Verification items for the finished model (mm, model axes). Face numbers are marked on the shaded views. A direction names the side the tool comes from. Round coordinates to 2 decimals unless told otherwise and drop trailing zeros. Order: outer loops, then holes, each group sorted by start corner. A loop starts at its lowest first (then second) coordinate and runs counter-clockwise, first axis right, second up. Notation, with made-up numbers: (73, -31.75) -> (113, -31.75) arc R17 ccw to (113, 0.25) -> close; hole circle Ø9 at (12, 82.25). An arc over 180 degrees is marked (long way). Answer in a Markdown table with one row per item. Add a question column.
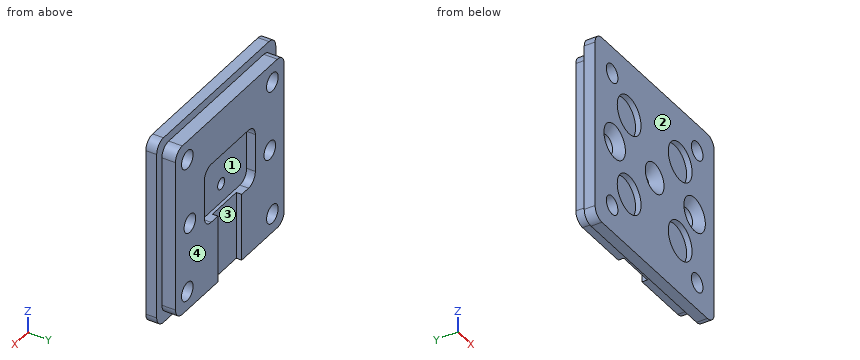
```python
from build123d import *

# Parameters (mm, degrees)
EXTRUDE_1_DEPTH              = 2.5
EXTRUDE_2_DEPTH              = 2
HOLE_WIZARD_3_4_D            = 3.4
CUT_EXTRUDE_2193_DEPTH       = 1.6
HOLE_WIZARD_3_D              = 3.4
HOLE_WIZARD_3_CSINK_D        = 6.3
HOLE_WIZARD_3_CSINK_ANGLE    = 90
SKETCH_8_W                   = 7
SKETCH_8_H                   = 12.475
CUT_EXTRUDE_3485_DEPTH       = 1
SKETCH_11_R                  = 3.5
CUT_EXTRUDE_7_1_DEPTH        = 1
HOLE_WIZARD_M2_5_D           = 2.05
HOLE_WIZARD_M2_5_CSINK_D     = 5.5
HOLE_WIZARD_M2_5_CSINK_ANGLE = 90


with BuildPart() as part:
    # Эскиз1 → Бобышка-Вытянуть1 (new body)
    with BuildSketch(Plane(origin=(0, 0, 0), x_dir=(1, 0, 0), z_dir=(0, 1, 0))):
        with BuildLine():
            Line((-13.975, 15.975), (13.975, 15.975))
            ThreePointArc((13.975, 15.975), (15.389213562, 15.389213562), (15.975, 13.975))
            Line((15.975, 13.975), (15.975, -13.975))
            ThreePointArc((15.975, -13.975), (15.389213562, -15.389213562), (13.975, -15.975))
            Line((13.975, -15.975), (-13.975, -15.975))
            ThreePointArc((-13.975, -15.975), (-15.389213562, -15.389213562), (-15.975, -13.975))
            Line((-15.975, -13.975), (-15.975, 13.975))
            ThreePointArc((-15.975, 13.975), (-15.389213562, 15.389213562), (-13.975, 15.975))
        make_face()
    extrude(amount=EXTRUDE_1_DEPTH)

    # Эскиз9 → Бобышка-Вытянуть2 (add)
    with BuildSketch(Plane.XZ):
        with BuildLine():
            Line((-15.5, 17.5), (15.5, 17.5))
            ThreePointArc((15.5, 17.5), (16.914213562, 16.914213562), (17.5, 15.5))
            Line((17.5, 15.5), (17.5, -15.5))
            ThreePointArc((17.5, -15.5), (16.914213562, -16.914213562), (15.5, -17.5))
            Line((15.5, -17.5), (-15.5, -17.5))
            ThreePointArc((-15.5, -17.5), (-16.914213562, -16.914213562), (-17.5, -15.5))
            Line((-17.5, -15.5), (-17.5, 15.5))
            ThreePointArc((-17.5, 15.5), (-16.914213562, 16.914213562), (-15.5, 17.5))
        make_face()
    extrude(amount=EXTRUDE_2_DEPTH)

    # Диаметр отверстия Ø3.4 (through all)
    with Locations(Plane.XZ.offset(2)):
        with Locations((-12.5, -12.5), (12.5, -12.5), (12.5, 12.5), (-12.5, 12.5)):
            Hole(HOLE_WIZARD_3_4_D / 2)

    # Эскиз4 → Cut-Extrude 2193 (cut)
    with BuildSketch(Plane(origin=(0, 2.5, 0), x_dir=(1, 0, 0), z_dir=(0, 1, 0))):
        with BuildLine():
            Line((-5.5, 3.5), (5.5, 3.5))
            ThreePointArc((5.5, 3.5), (6.914213562, 2.914213562), (7.5, 1.5))
            Line((7.5, 1.5), (7.5, -5.5))
            ThreePointArc((7.5, -5.5), (6.914213562, -6.914213562), (5.5, -7.5))
            Line((5.5, -7.5), (-5.5, -7.5))
            ThreePointArc((-5.5, -7.5), (-6.914213562, -6.914213562), (-7.5, -5.5))
            Line((-7.5, -5.5), (-7.5, 1.5))
            ThreePointArc((-7.5, 1.5), (-6.914213562, 2.914213562), (-5.5, 3.5))
        make_face()
    extrude(amount=-CUT_EXTRUDE_2193_DEPTH, mode=Mode.SUBTRACT)

    # Крепление дна М3 (through all)
    with Locations(Plane(origin=(0, -2, 0), x_dir=(-1, 0, 0), z_dir=(0, -1, 0))):
        with Locations((11.75, 0), (-11.75, 0)):
            CounterSinkHole(HOLE_WIZARD_3_D / 2, HOLE_WIZARD_3_CSINK_D / 2, counter_sink_angle=HOLE_WIZARD_3_CSINK_ANGLE)

    # Эскиз8 → Cut-Extrude 3485 (cut)
    with BuildSketch(Plane(origin=(0, 2.5, 0), x_dir=(1, 0, 0), z_dir=(0, 1, 0))):
        with Locations((0, 9.7375)):
            Rectangle(SKETCH_8_W, SKETCH_8_H)
    extrude(amount=-CUT_EXTRUDE_3485_DEPTH, mode=Mode.SUBTRACT)

    # Эскиз11 → Вырез магнитов 7*1 (cut)
    with BuildSketch(Plane.XZ.offset(2)):
        with Locations(Location((-7.5, 7.5, 0), (0, 0, 270))):
            Circle(SKETCH_11_R)
        with Locations(Location((7.5, 7.5, 0), (0, 0, 270))):
            Circle(SKETCH_11_R)
        with Locations(Location((-7.5, -7.5, 0), (0, 0, 270))):
            Circle(SKETCH_11_R)
        with Locations(Location((7.5, -7.5, 0), (0, 0, 270))):
            Circle(SKETCH_11_R)
    extrude(amount=-CUT_EXTRUDE_7_1_DEPTH, mode=Mode.SUBTRACT)

    # Отверстие для настройки M2.5 (through all)
    with Locations(Plane(origin=(0, -2, 0), x_dir=(-1, 0, 0), z_dir=(0, -1, 0))):
        with Locations((0, 0)):
            CounterSinkHole(HOLE_WIZARD_M2_5_D / 2, HOLE_WIZARD_M2_5_CSINK_D / 2, counter_sink_angle=HOLE_WIZARD_M2_5_CSINK_ANGLE)


solid = part.part
```
1) Cross-section at C-C, the plane z = -12.5. Record the boundary of the cut face in (x, y) (3 decimals).
2) Draft check along X on the marked faces 3 and 4. Enter one of: +X half, -X half, draft (parallel to the pull), parting line (faces both ways), or undercut.
3) Tool access check on the marked faces 1 and 2. Record the directions out of +Z, -Z, +X, -X, +Y, -Y that give a thin tool (end or side, any length) a straight path to the whole face; none if there is none.
4) Thickness scan on L1, parallel to X at y = -1.7, z = -7.5; L2, parallel to Z at x = 5, y = 1.1 (3 decimals); L3, parallel to X at y = -1.75, z = -4.5. Record the ranges inside material, lowest first. Write a range as [from, to].
5) Depth check by flat-ended pin: P1, Ø11, axis at x = -7.5, z = 7.5, coming from the -Y side; P2, Ø0.5, axis at y = 1.5, z = 3.5, coming from the +X side (3 decimals); P3, Ø0.8, axis at y = 2, z = 2, coming from the -X side (3 decimals); P4, Ø0.5, axis at x = -0.5, y = 2, coming from the -Z side. Enter the tip coordinate at first touch or a pass-through.
6) Cross-section at D-D, the plane x = 11.75. Record the boundary of the cut face in (y, z) (3 decimals), and give its area (3 significant figures).
7) Cross-section at A-A, the plane x = 0. Record the boundary of the cut face in (y, z) (3 decimals), and give its area (3 significant figures).
8) Cross-section at B-B, the plane y = -1.55. Give the number of separate pieces and of enclosed holes in the cut face, and give its area (3 significant figures).
Results below:
| question | item | result |
|---|---|---|
| 1 | outline | (-17.5, -2) -> (-14.2, -2) -> (-14.2, 2.5) -> (-15.975, 2.5) -> (-15.975, 0) -> (-17.5, 0) -> close; (-10.8, -2) -> (10.8, -2) -> (10.8, 2.5) -> (3.5, 2.5) -> (3.5, 1.5) -> (-3.5, 1.5) -> (-3.5, 2.5) -> (-10.8, 2.5) -> close; (14.2, -2) -> (17.5, -2) -> (17.5, 0) -> (15.975, 0) -> (15.975, 2.5) -> (14.2, 2.5) -> close |
| 2 | face 3 | undercut |
| 2 | face 4 | draft |
| 3 | face 1 | +Y |
| 3 | face 2 | +Z, -Z, +X, -X, -Y |
| 4 | L1 | [-17.5, -11], [-4, 4], [11, 17.5] |
| 4 | L2 | [-15.975, -3.5], [7.5, 15.975] |
| 4 | L3 | [-17.5, -9.3], [-5.7, 5.7], [9.3, 17.5] |
| 5 | P1 | y = -2 |
| 5 | P2 | x = 15.975 |
| 5 | P3 | x = -15.975 |
| 5 | P4 | z = 7.5 |
| 6 | outline | (-2, -17.5) -> (0, -17.5) -> (0, -15.975) -> (2.5, -15.975) -> (2.5, -14.026) -> (-2, -14.026) -> close; (-2, -10.974) -> (2.5, -10.974) -> (2.5, -1.7) -> (-0.55, -1.7) -> (-2, -3.15) -> close; (-2, 3.15) -> (-0.55, 1.7) -> (2.5, 1.7) -> (2.5, 10.974) -> (-2, 10.974) -> close; (-2, 14.026) -> (2.5, 14.026) -> (2.5, 15.975) -> (0, 15.975) -> (0, 17.5) -> (-2, 17.5) -> close |
| 6 | area | 105 mm² |
| 7 | outline | (-2, -17.5) -> (0, -17.5) -> (0, -15.975) -> (1.5, -15.975) -> (1.5, -3.5) -> (0.9, -3.5) -> (0.9, -1.025) -> (-0.275, -1.025) -> (-2, -2.75) -> close; (-2, 2.75) -> (-0.275, 1.025) -> (0.9, 1.025) -> (0.9, 7.5) -> (2.5, 7.5) -> (2.5, 15.975) -> (0, 15.975) -> (0, 17.5) -> (-2, 17.5) -> close |
| 7 | area | 111 mm² |
| 8 | separate pieces | 1 |
| 8 | enclosed holes | 11 |
| 8 | area | 969 mm² |
